Read the model definition and answer for the solid it produces. Units are mm, in the model's axes. A direction names the side the tool comes from. Give positions to 0.01 mm unless a question says otherwise; leave off trailing zeros. Loops run counter-clockwise (first coordinate to the right, second up) from the corner with the lowest first, then second, coordinate; pieces in that order, holes last. Notation, with made-up numbers: M 82,22.25 L 141,22.25 A24 cw 141,45.25 Z; hole C 76,53 d8. An arc over 180 degrees is marked long. Return JSON: item names as keys, results as strings. Group by question number.
Autodesk Inventor part; units mm, degrees
ref_plane "YZ Plane" through (0, 0, 0) normal (1, 0, 0) x (0, 1, 0)
ref_plane "XZ Plane" through (0, 0, 0) normal (0, 1, 0) x (-1, 0, 0)
ref_plane "XY Plane" through (0, 0, 0) normal (0, 0, 1) x (1, 0, 0)
sketch "Sketch1" plane through (0, 0, 0) normal (0, 1, 0) x (-1, 0, 0)
  line L0 (0, 0) -> (101.6, 0)
  line L1 (101.6, 0) -> (101.6, 25.4)
  line L2 (101.6, 25.4) -> (0, 25.4)
  line L3 (0, 25.4) -> (0, 0)
  dimension "d0" = 101.6
  dimension "d1" = 25.4
extrude "Extrusion1" add sketch "Sketch1" along normal blind 50.8
sketch "Sketch2" plane through (-101.6, 0, 25.4) normal (0, 0, 1) x (1, 0, 0)
  circle A0 centre (25.4, 19.05) radius 7.9375
  line L0 (101.6, 50.8) -> (0, 50.8)
  line L1 (101.6, 0) -> (101.6, 50.8)
  dimension "d4" = 15.875
  dimension "d5" = 31.75
  dimension "d6" = 76.2
extrude "Extrusion2" cut sketch "Sketch2" against normal blind 111.125
sketch "Sketch3" plane through (0, 0, 25.4) normal (1, 0, 0) x (0, 0, -1)
  line L0 (3.175, 3.175) -> (22.225, 3.175)
  line L1 (22.225, 3.175) -> (22.225, 47.625)
  line L2 (22.225, 47.625) -> (3.175, 47.625)
  line L3 (3.175, 47.625) -> (3.175, 3.175)
  line L4 (0, 0) -> (0, 50.8)
  line L5 (0, 0) -> (25.4, 0)
  line L6 (25.4, 0) -> (25.4, 50.8)
  line L7 (25.4, 50.8) -> (0, 50.8)
  dimension "d9" = 3.175
  dimension "d10" = 3.175
  dimension "d11" = 3.175
  dimension "d12" = 3.175
extrude "Extrusion3" cut sketch "Sketch3" against normal blind 111.125 contours L3 L2 L1 L0
sketch "Sketch4" plane through (0, 50.8, 0) normal (0, 1, 0) x (1, 0, 0)
  circle A0 centre (-12.7, -12.827) radius 2.54
  circle A1 centre (-88.9, -12.827) radius 2.54
  line L0 (0, 0) -> (-101.6, 0)
  line L1 (-101.6, 0) -> (-101.6, -25.4)
  line L2 (0, -25.4) -> (0, 0)
  dimension "d15" = 5.08
  dimension "d16" = 12.827
  dimension "d17" = 12.7
  dimension "d18" = 5.08
  dimension "d19" = 12.827
  dimension "d20" = 12.7
  dimension "d21" = 76.2
extrude "Extrusion4" cut sketch "Sketch4" against normal blind 111.125
sketch "Sketch5" plane through (-101.6, 0, 25.4) normal (0, 0, 1) x (1, 0, 0)
  circle A0 centre (25.4, 19.05) radius 7.9375
  circle A1 centre (25.4, 19.05) radius 14.2875
  point P0 (101.6, 0)
  dimension "d24" = 28.575
extrude "Extrusion5" cut sketch "Sketch5" against normal blind 5.08
properties part number "15102898-16-P-0306" material "Aluminum 6061"
1. Find section B-B (x = -76.2). Write down the section's boundary in (y, z) (1 decimal).
2. Find section C-C (y = 19.05). Write down the section's boundary in (x, z) (1 decimal), and give its area (3 significant figures).
3. Straight lines are drawn through the part: line 1 along Z through (x, y) = (-88.9, 2.55); line 2 along Z through (x, y) = (-83.5, 40) (3 decimals); line 3 along Y through (x, z) = (-96, 20.5) (3 decimals). For each, find the intervals that lie inside material, in ascending order.
4. The mould has two halves that part along X. Classify faces 1 (the flat face through (-50, 47.625, 13)), 2 (the cylindrical face through (-14.72, 49.23, 14.37)), 3 (the flat face through (-101.6, 27, 2)), 4 (the flat face through (0, 27, 23)): +X half, -X half, draft (parallel to the pull), parting line (faces both ways), or undercut.
5. For faces 5 (the cylindrical face through (-86.554, 49.235, 13.8)), 6 (the flat face through (-50, 26, 22.225)), 7 (the cylindrical face through (-90.474, 19.678, 23.835)), determine the directions among +Z, -Z, +X, -X, +Y, -Y from which every point of the face is accessible in a straight line to the end or side of a thin tool.
6. A flat-ended cylindrical pin translates along its axis: P1, Ø18.5, axis at x = -76.2, y = 19.05, coming from the +Z side (3 decimals). Find the tip coordinate at first contact, or state that the pin passes through.
7. Find section A-A (z = 16.5). Write down the section's boundary in (x, y) (3 decimals).
8. Find section D-D (x = -50.5). Write down the section's boundary in (y, z) (3 decimals), and give its area (3 significant figures).
Result:
{
 "1": {"outline": "M 0,0 L 11.1,0 L 11.1,3.2 L 3.2,3.2 L 3.2,22.2 L 4.8,22.2 L 4.8,25.4 L 0,25.4 Z; M 27,0 L 50.8,0 L 50.8,25.4 L 33.3,25.4 L 33.3,22.2 L 47.6,22.2 L 47.6,3.2 L 27,3.2 Z"},
 "2": {"outline": "M -101.6,0 L -84.1,0 L -84.1,3.2 L -101.6,3.2 Z; M -101.6,22.2 L -90.5,22.2 L -90.5,25.4 L -101.6,25.4 Z; M -68.3,0 L 0,0 L 0,3.2 L -68.3,3.2 Z; M -61.9,22.2 L 0,22.2 L 0,25.4 L -61.9,25.4 Z", "area": "504 mm2"},
 "3": {"line 1": "z = 0 to 10.29, 15.37 to 25.4", "line 2": "z = 0 to 3.175, 22.225 to 25.4", "line 3": "y = 0 to 3.175, 47.625 to 50.8"},
 "4": {"face 1": "draft", "face 2": "undercut", "face 3": "-X half", "face 4": "+X half"},
 "5": {"face 5": "+Y, -Y", "face 6": "+X, -X", "face 7": "+Z"},
 "6": {"P1": "stops at z = 3.175"},
 "7": {"outline": "M -101.6,0 L 0,0 L 0,3.175 L -101.6,3.175 Z; M -101.6,47.625 L 0,47.625 L 0,50.8 L -101.6,50.8 Z"},
 "8": {"outline": "M 0,0 L 50.8,0 L 50.8,25.4 L 0,25.4 Z; hole M 3.175,3.175 L 47.625,3.175 L 47.625,22.225 L 3.175,22.225 Z", "area": "444 mm2"}
}
